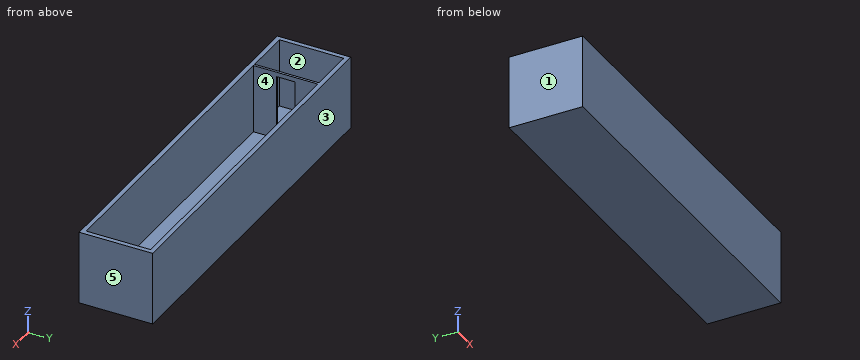
from build123d import *

# Parameters (mm, degrees)
F0_W          = 101.6
F0_H          = 20.32
F1_DEPTH      = 10.16
F1_DEPTH_BACK = 10.16
F2_W          = 99.06
F2_H          = 17.78
F3_DEPTH      = 19.05
F4_W          = 0.635
F4_H          = 6.35
F5_DEPTH      = 19.05
F6_START      = 17.78
F4_H_2        = 5.08
F6_DEPTH      = 1.27


with BuildPart() as f1:
    # F0 (on Front) → F1 (new body, two sides)
    with BuildSketch(Plane.XZ) as f1_sk:
        Rectangle(F0_W, F0_H)
    extrude(amount=F1_DEPTH)
    extrude(f1_sk.sketch, amount=-F1_DEPTH_BACK)

    # F2 (on face) → F3 (cut)
    with BuildSketch(Plane.XY.offset(10.16)):
        Rectangle(F2_W, F2_H)
    extrude(amount=-F3_DEPTH, mode=Mode.SUBTRACT)

    # F4 (on face) → F5 (join)
    with BuildSketch(Plane.XY.offset(-8.89)):
        with Locations((-36.5125, -5.715)):
            Rectangle(F4_W, F4_H)
        with Locations((-36.5125, 5.715)):
            Rectangle(F4_W, F4_H)
    extrude(amount=F5_DEPTH)

    # F4 (on face) → F6 (join)
    with BuildSketch(Plane.XY.offset(-8.89).offset(F6_START)):
        with Locations((-36.5125, 0)):
            Rectangle(F4_W, F4_H_2)
    extrude(amount=F6_DEPTH)


solid = f1.part
Input: part model. Units: mm. Frame: model coordinates. Face numbers are marked on the shaded views. A direction names the side the tool comes from. Round coordinates to 2 decimals unless told otherwise and drop trailing zeros. Order: outer loops, then holes, each group sorted by start corner. A loop starts at its lowest first (then second) coordinate and runs counter-clockwise, first axis right, second up. Notation, with made-up numbers: (24.5, 42.5) - (82.5, 42.5) arc R10 ccw to (82.5, 53.5) - close; hole circle Ø8 at (15.5, 60.25). An arc over 180 degrees is marked (long way). Use a Markdown table: item, result.
1. First-contact query: pin 1 (8 mm diameter, centred on x = 30, y = 4.5, fed in from +Z). Flat tip, straight axial feed; report the tip coordinate or a pass-through.
Evaluation:
| item | result |
|---|---|
| pin 1 | z = -8.89 |
2. Section B-B on z = 2.5. Return the cut outline in (x, y) (3 decimals).
Evaluation:
| item | result |
|---|---|
| outline | (-50.8, -10.16) - (50.8, -10.16) - (50.8, 10.16) - (-50.8, 10.16) - close; hole (-49.53, -8.89) - (-36.83, -8.89) - (-36.83, -2.54) - (-36.195, -2.54) - (-36.195, -8.89) - (49.53, -8.89) - (49.53, 8.89) - (-36.195, 8.89) - (-36.195, 2.54) - (-36.83, 2.54) - (-36.83, 8.89) - (-49.53, 8.89) - close |
3. Section D-D on x = 41. Return the cut outline in (y, z), then the cut area to 3 significant figures.
Evaluation:
| item | result |
|---|---|
| outline | (-10.16, -10.16) - (10.16, -10.16) - (10.16, 10.16) - (8.89, 10.16) - (8.89, -8.89) - (-8.89, -8.89) - (-8.89, 10.16) - (-10.16, 10.16) - close |
| area | 74.2 mm^2 |
4. Section C-C on y = -5. Return the cut outline in (x, z) (3 decimals), then the cut area to 3 significant figures.
Evaluation:
| item | result |
|---|---|
| outline | (-50.8, -10.16) - (50.8, -10.16) - (50.8, 10.16) - (49.53, 10.16) - (49.53, -8.89) - (-36.195, -8.89) - (-36.195, 10.16) - (-36.83, 10.16) - (-36.83, -8.89) - (-49.53, -8.89) - (-49.53, 10.16) - (-50.8, 10.16) - close |
| area | 190 mm^2 |
5. Mould query, pull axis X, two halves, no side actions, for the marked faces 1, 2 and 3. Classes: +X half, -X half, draft (parallel to the pull), parting line (faces both ways), or undercut.
Evaluation:
| item | result |
|---|---|
| face 1 | -X half |
| face 2 | undercut |
| face 3 | draft |
6. Access query for the marked faces 4 and 5. Directions: +Z, -Z, +X, -X, +Y, -Y. A direction counts if a zero-diameter tool reaches every point of the face in a straight line with its end or side. Return the directions, or none.
Evaluation:
| item | result |
|---|---|
| face 4 | +Z |
| face 5 | +Z, -Z, +X, +Y, -Y |
7. Material intervals for probe 1 along X at (y, z) = (-5, -1) (3 decimals); probe 2 along Y at (x, z) = (-28, -2); probe 3 along X at (y, z) = (0.5, 8), sorted ascending.
Evaluation:
| item | result |
|---|---|
| probe 1 | -50.8 to -49.53, -36.83 to -36.195, 49.53 to 50.8 |
| probe 2 | -10.16 to -8.89, 8.89 to 10.16 |
| probe 3 | -50.8 to -49.53, 49.53 to 50.8 |
8. Section A-A on y = -0.5. Return the cut outline in (x, z) (3 decimals), then the cut area to 3 significant figures.
Evaluation:
| item | result |
|---|---|
| outline | (-50.8, -10.16) - (50.8, -10.16) - (50.8, 10.16) - (49.53, 10.16) - (49.53, -8.89) - (-49.53, -8.89) - (-49.53, 10.16) - (-50.8, 10.16) - close; (-36.83, 8.89) - (-36.195, 8.89) - (-36.195, 10.16) - (-36.83, 10.16) - close |
| area | 178 mm^2 |
